```python
from build123d import *

# Parameters (mm, degrees)
F1_DEPTH       = 15
F2_R           = 3
F4_D           = 4
F4_CSINK_D     = 8
F4_CSINK_ANGLE = 90
F5_R           = 4


with BuildPart() as f1:
    # F0 (on Top) → F1 (new body)
    with BuildSketch(Plane.XY):
        with BuildLine():
            Line((20.835556, 37.046353), (20.835556, 29.997582))
            Line((20.835556, 29.997582), (101.955885, 29.997582))
            Line((101.955885, 29.997582), (101.955885, 37.046353))
            Line((101.955885, 37.046353), (75.967759, 37.046353))
            ThreePointArc((75.967759, 37.046353), (89.452061, 57.015966), (82.430315, 80.066062))
            Line((82.430315, 80.066062), (82.492916, 80.06982))
            Line((82.492916, 80.06982), (82.492916, 85.78659))
            Line((82.492916, 85.78659), (75.115513, 85.78659))
            Line((75.115513, 85.78659), (75.732713, 79.446834))
            ThreePointArc((75.732713, 79.446834), (61.595594, 38.176149), (48.059836, 79.647957))
            Line((48.059836, 79.647957), (48.409987, 85.78659))
            Line((48.409987, 85.78659), (41.504001, 85.78659))
            Line((41.504001, 85.78659), (41.504001, 80.503838))
            ThreePointArc((41.504001, 80.503838), (33.996464, 57.565367), (47.120148, 37.309369))
            ThreePointArc((47.120148, 37.309369), (47.338346, 37.176863), (47.557742, 37.046353))
            Line((47.557742, 37.046353), (20.835556, 37.046353))
        make_face()
    extrude(amount=F1_DEPTH)

    # F2
    f2_edges = [f1.edges().sort_by_distance(p)[0] for p in [
        (75.115513, 85.78659, 7.5),
        (82.492916, 85.78659, 7.5),
        (48.409987, 85.78659, 7.5),
        (41.504001, 85.78659, 7.5),
        (20.835556, 37.046353, 7.5),
        (101.955885, 37.046353, 7.5),
    ]]
    fillet(f2_edges, radius=F2_R)

    # F4 (through all)
    with Locations(Plane(origin=(0, 37.046353, 0), x_dir=(-1, 0, 0), z_dir=(0, 1, 0))):
        with Locations((-94.379296, 7.332574), (-28.848284, 7.332574)):
            CounterSinkHole(F4_D / 2, F4_CSINK_D / 2, counter_sink_angle=F4_CSINK_ANGLE)

    # F5
    f5_edges = [f1.edges().sort_by_distance(p)[0] for p in [
        (75.967759, 37.046353, 7.5),
        (47.557742, 37.046353, 7.5),
    ]]
    fillet(f5_edges, radius=F5_R)


solid = f1.part
```
Input: part model. Units: mm. Frame: model coordinates. A direction names the side the tool comes from. Coordinates: 2 decimals unless noted, no trailing zeros. Loops run counter-clockwise (first coordinate to the right, second up) from the corner with the lowest first, then second, coordinate; pieces in that order, holes last. Notation, with made-up numbers: M 38,35.25 L 78,35.25 A29 ccw 78,61.25 Z; hole C 13,51.25 d10. An arc over 180 degrees is marked long. Answer in a Markdown table with one row per item.
1. Section A-A, the plane y = 52. Output: boundary loops of the cut face in (x, z), then the cut area to 3 significant figures.
Response:
| item | result |
|---|---|
| outline | M 35.31,0 L 40.67,0 L 40.67,15 L 35.31,15 Z; M 82.85,0 L 88.22,0 L 88.22,15 L 82.85,15 Z |
| area | 161 mm2 |
2. First-contact query: pin 1 (0.8 mm diameter, centred on y = 81.5, z = 9.5, fed in from +X); pin 2 (1.5 mm diameter, centred on y = 53.5, z = 8.5, fed in from +X); pin 3 (1.8 mm diameter, centred on y = 81, z = 9.5, fed in from -X). Flat tips, straight axial feed; report the tip coordinate or a pass-through.
Response:
| item | result |
|---|---|
| pin 1 | stops at x = 82.49 |
| pin 2 | stops at x = 88.89 |
| pin 3 | stops at x = 41.13 |
3. Section C-C, the plane x = 55. Output: boundary loops of the cut face in (y, z).
Response:
| item | result |
|---|---|
| outline | M 30,0 L 39.19,0 L 39.19,15 L 30,15 Z |
4. Section B-B, the plane y = 70.5. Output: boundary loops of the cut face in (x, z).
Response:
| item | result |
|---|---|
| outline | M 35.36,0 L 40.74,0 L 40.74,15 L 35.36,15 Z; M 82.79,0 L 88.16,0 L 88.16,15 L 82.79,15 Z |
5. Draft query along Y for faces 4 (the flat face through (61, 29.998, 7)), 5 (the flat face through (90, 37.046, 7)), 6 (the cylindrical face through (42.406, 84.931, 7.605)), 7 (the flat face through (75.582, 80.993, 7.395)). Return one class per face: pulls with the +Y half, pulls with the -Y half, needs draft (parallel to the pull), parting line crosses it, or undercut.
Response:
| item | result |
|---|---|
| face 4 | pulls with the -Y half |
| face 5 | undercut |
| face 6 | pulls with the +Y half |
| face 7 | undercut |
6. Section D-D, the plane x = 68.5. Output: boundary loops of the cut face in (y, z).
Response:
| item | result |
|---|---|
| outline | M 30,0 L 39.18,0 L 39.18,15 L 30,15 Z |
7. Material intervals for line 1 (Y direction, x = 36, z = 12); line 2 (X direction, y = 33, z = 9); line 3 (X direction, y = 63, z = 4.5), sorted ascending.
Response:
| item | result |
|---|---|
| line 1 | y = 30 to 37.05, 50.21 to 72.14 |
| line 2 | x = 20.84 to 27.74, 29.95 to 93.27, 95.48 to 101.96 |
| line 3 | x = 33.82 to 38.84, 84.69 to 89.7 |
8. Reachability of faces 1 (the flat face through (33, 37.046, 7)), 2 (the flat face through (58, 37, 0)), 3 (the flat face through (82.493, 81, 7)) from +Z, -Z, +X, -X, +Y, -Y: full face, straight path, thin tool, end or side. Return the list, or none.
Response:
| item | result |
|---|---|
| face 1 | +Z, -Z, -X |
| face 2 | -Z, +X, -X, +Y, -Y |
| face 3 | +Z, -Z, +X, +Y |
